Autodesk Inventor part; units mm, degrees
ref_plane "YZ Plane" through (0, 0, 0) normal (1, 0, 0) x (0, 1, 0)
ref_plane "XZ Plane" through (0, 0, 0) normal (0, 1, 0) x (-1, 0, 0)
ref_plane "XY Plane" through (0, 0, 0) normal (0, 0, 1) x (1, 0, 0)
sketch "Sketch1" plane through (0, 0, 0) normal (0, 0, 1) x (1, 0, 0)
  line L0 (-40, 42.5) -> (40, 42.5)
  line L1 (40, 42.5) -> (40, -42.5)
  line L2 (40, -42.5) -> (-40, -42.5)
  line L3 (-40, -42.5) -> (-40, 42.5)
  line L4 (-40, 42.5) -> (40, -42.5) construction
  line L5 (40, 42.5) -> (-40, -42.5) construction
  line L6 (40, 42.5) -> (30, 42.5)
  line L7 (30, 42.5) -> (30, 52.5)
  line L8 (30, 52.5) -> (40, 52.5)
  line L9 (40, 52.5) -> (40, 42.5)
  line L10 (-40, 42.5) -> (-30, 42.5)
  line L11 (-30, 42.5) -> (-30, 52.5)
  line L12 (-30, 52.5) -> (-40, 52.5)
  line L13 (-40, 52.5) -> (-40, 42.5)
  line L14 (-40, -42.5) -> (-30, -42.5)
  line L15 (-30, -42.5) -> (-30, -52.5)
  line L16 (-30, -52.5) -> (-40, -52.5)
  line L17 (-40, -52.5) -> (-40, -42.5)
  line L18 (40, -42.5) -> (30, -42.5)
  line L19 (30, -42.5) -> (30, -52.5)
  line L20 (30, -52.5) -> (40, -52.5)
  line L21 (40, -52.5) -> (40, -42.5)
  circle A0 centre (-35, 47.5) radius 2.75
  circle A1 centre (35, 47.5) radius 2.75
  circle A2 centre (35, -47.5) radius 2.75
  circle A3 centre (-35, -47.5) radius 2.75
  point P0 (0, 0)
  point P1 (-35, 52.5)
  point P2 (35, 52.5)
  point P3 (-40, -47.5)
  point P4 (-40, 47.5)
  point P5 (30, -42.5)
  point P6 (30, 42.5)
  point P7 (30, -47.5)
  dimension "d1" = 10
  dimension "d2" = 10
  dimension "d3" = 5.5
  dimension "d4" = 5.5
  dimension "d5" = 5.5
  dimension "d6" = 5.5
  dimension "d7" = 10
  dimension "d8" = 10
  dimension "d9" = 85
  dimension "d10" = 80
extrude "Extrusion1" add sketch "Sketch1" along normal blind 10
sketch "Sketch2" plane through (0, 0, 10) normal (0, 0, 1) x (1, 0, 0)
  circle A0 centre (-30, 32.5) radius 5
  line L0 (-40, 52.5) -> (-40, -52.5)
  line L1 (30, 42.5) -> (-30, 42.5)
  circle A1 centre (-15, 32.5) radius 5
  circle A2 centre (0, 32.5) radius 5
  circle A3 centre (15, 32.5) radius 5
  circle A4 centre (30, 32.5) radius 5
  circle A5 centre (-30, 16.5) radius 5
  circle A6 centre (-15, 16.5) radius 5
  circle A7 centre (0, 16.5) radius 5
  circle A8 centre (15, 16.5) radius 5
  circle A9 centre (30, 16.5) radius 5
  circle A10 centre (-30, 0.5) radius 5
  circle A11 centre (-15, 0.5) radius 5
  circle A12 centre (0, 0.5) radius 5
  circle A13 centre (15, 0.5) radius 5
  circle A14 centre (30, 0.5) radius 5
  circle A15 centre (-30, -15.5) radius 5
  circle A16 centre (-15, -15.5) radius 5
  circle A17 centre (0, -15.5) radius 5
  circle A18 centre (15, -15.5) radius 5
  circle A19 centre (30, -15.5) radius 5
  circle A20 centre (-30, -31.5) radius 5
  circle A21 centre (-15, -31.5) radius 5
  circle A22 centre (0, -31.5) radius 5
  circle A23 centre (15, -31.5) radius 5
  circle A24 centre (30, -31.5) radius 5
  point P0 (0, 0)
  dimension "d13" = 10
  dimension "d14" = 10
  dimension "d15" = 10
  dimension "d18" = 15
  dimension "d21" = 16
extrude "Extrusion2" cut sketch "Sketch2" against normal blind 10
properties part number "battery_box_cap_ver2"
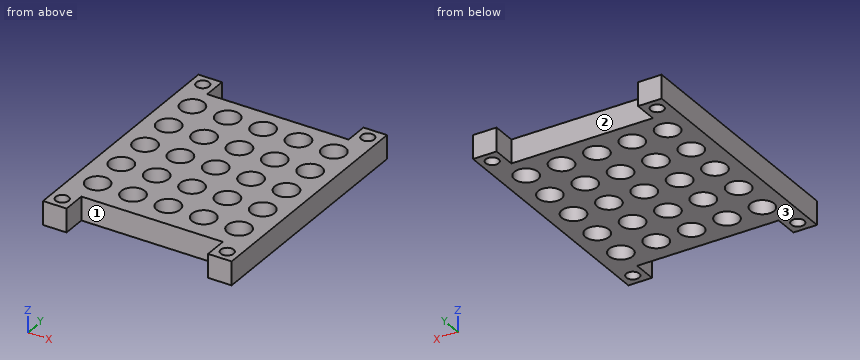
Part model, mm, in its own coordinate system. Face numbers are marked on the shaded views. A direction names the side the tool comes from. Round coordinates to 2 decimals unless told otherwise and drop trailing zeros. Loops run counter-clockwise (first coordinate to the right, second up) from the corner with the lowest first, then second, coordinate; pieces in that order, holes last. Notation, with made-up numbers: (53, -3) -> (61, -3) arc R31 cw to (61, 33) -> close; hole circle Ø7 at (58, 84). An arc over 180 degrees is marked (long way). Use one line per item in the form item = value. Start each with the question number.
Item 1: Tool access for the marked faces 1, 2 and 3: list every direction of +Z, -Z, +X, -X, +Y, -Y with a clear straight run to the whole face (end or side of a thin tool).
Item 2: Band-saw the part on C-C (y = 0.5). List the corners of the cut face in (x, z), plus the area to 3 significant figures.
Item 3: Band-saw the part on D-D (z = 8). Give the number of separate pieces and of enclosed holes in the cut face, plus the area to 3 significant figures.
Item 4: Band-saw the part on A-A (x = -15). List the corners of the cut face in (y, z), plus the area to 3 significant figures.
Item 5: Drop flat-ended pins along their axis: pin 1 Ø8 at (x, y) = (-30, 0.5) entering from +Z; pin 2 Ø1.5 at (x, z) = (-20, 4.5) entering from +Y. Give the stop position or say it passes through.
Item 6: Drill centre lines: line 1 along Y through (x, z) = (-15, 5.5); line 2 along X through (y, z) = (-15, 4.75); line 3 along Y through (x, z) = (-16, 3.25). Where is each one in solid material? Low to high.
Item 7: Band-saw the part on B-B (y = 47.5). List the corners of the cut face in (x, z), plus the area to 3 significant figures.
Data:
q1.face_1 = +Z, -Z, -Y
q1.face_2 = +Z, -Z, +Y
q1.face_3 = -Z, +X, -X, +Y, -Y
q2.outline = (-40, 0) -> (-35, 0) -> (-35, 10) -> (-40, 10) -> close; (-25, 0) -> (-20, 0) -> (-20, 10) -> (-25, 10) -> close; (-10, 0) -> (-5, 0) -> (-5, 10) -> (-10, 10) -> close; (5, 0) -> (10, 0) -> (10, 10) -> (5, 10) -> close; (20, 0) -> (25, 0) -> (25, 10) -> (20, 10) -> close; (35, 0) -> (40, 0) -> (40, 10) -> (35, 10) -> close
q2.area = 300 mm^2
q3.separate_pieces = 1
q3.enclosed_holes = 29
q3.area = 5,140 mm^2
q4.outline = (-42.5, 0) -> (-36.5, 0) -> (-36.5, 10) -> (-42.5, 10) -> close; (-26.5, 0) -> (-20.5, 0) -> (-20.5, 10) -> (-26.5, 10) -> close; (-10.5, 0) -> (-4.5, 0) -> (-4.5, 10) -> (-10.5, 10) -> close; (5.5, 0) -> (11.5, 0) -> (11.5, 10) -> (5.5, 10) -> close; (21.5, 0) -> (27.5, 0) -> (27.5, 10) -> (21.5, 10) -> close; (37.5, 0) -> (42.5, 0) -> (42.5, 10) -> (37.5, 10) -> close
q4.area = 350 mm^2
q5.pin_1 = through
q5.pin_2 = 42.5
q6.line_1 = -42.5 to -36.5, -26.5 to -20.5, -10.5 to -4.5, 5.5 to 11.5, 21.5 to 27.5, 37.5 to 42.5
q6.line_2 = -40 to -34.97, -25.03 to -19.97, -10.03 to -4.97, 4.97 to 10.03, 19.97 to 25.03, 34.97 to 40
q6.line_3 = -42.5 to -36.4, -26.6 to -20.4, -10.6 to -4.4, 5.4 to 11.6, 21.4 to 27.6, 37.4 to 42.5
q7.outline = (-40, 0) -> (-37.75, 0) -> (-37.75, 10) -> (-40, 10) -> close; (-32.25, 0) -> (-30, 0) -> (-30, 10) -> (-32.25, 10) -> close; (30, 0) -> (32.25, 0) -> (32.25, 10) -> (30, 10) -> close; (37.75, 0) -> (40, 0) -> (40, 10) -> (37.75, 10) -> close
q7.area = 90.0 mm^2
